Here's how the part is built. I have some questions about the finished solid (model axes, mm). A direction names the side the tool comes from. Give positions to 0.01 mm unless a question says otherwise; leave off trailing zeros. Loops run counter-clockwise (first coordinate to the right, second up) from the corner with the lowest first, then second, coordinate; pieces in that order, holes last. Notation, with made-up numbers: (27.25, -25) -> (55.25, -25) arc R28 cw to (55.25, -7) -> close; hole circle Ø9 at (2.25, 49). An arc over 180 degrees is marked (long way). Answer in a Markdown table with one row per item. Add a question column.
Item 1: We'd pull the mould along X, two halves only. Please class faces 3 (the face through (72.227, -160.39, 4.696)), 4 (the face through (124, -168, 5)), 5 (the face through (131.89, -161.88, 4.7)), 6 (the face through (31, -203.2, 5)): released by +X, released by -X, zero draft, split by the parting line, or undercut.
Item 2: If I drill on line 1 (X direction, y = -141, z = 0.5); line 2 (X direction, y = -149.5, z = 1.5); line 3 (Y direction, x = 158, z = 6.5), over which ranges is the centre line in solid material (lowest first)?
Item 3: Which directions (+Z, -Z, +X, -X, +Y, -Y) give clear straight access to the entire face, cutting with the end or side of a thin tool? Please do faces 1 (the face through (172, -203.2, 5)), 2 (the face through (80.47, -166.26, 4.7)).
Item 4: If we section it at B-B (z = 5.75): Write out the boundary of the cut face in (x, y), then the cut area to 3 significant figures.
Item 5: For P1, Ø5, axis at x = 58.5, z = 1.5, coming from the +Y side; P2, Ø3, axis at y = -185.5, z = 7, coming from the -X side, each with a flat end and sliding along its axis, tell me the tip position at first contact or that it passes through.
Item 6: If we section it at A-A (y = -196): Write out the boundary of the cut face in (x, z) (3 decimals).
Item 7: If we section it at D-D (x = 127): Write out the boundary of the cut face in (y, z) (3 decimals), then the cut area to 3 significant figures.
Item 8: If we section it at C-C (y = -183): Write out the boundary of the cut face in (x, z) (3 decimals).
Autodesk Inventor part; units mm, degrees
ref_plane "YZ Plane" through (0, 0, 0) normal (1, 0, 0) x (0, 1, 0)
ref_plane "XZ Plane" through (0, 0, 0) normal (0, 1, 0) x (-1, 0, 0)
ref_plane "XY Plane" through (0, 0, 0) normal (0, 0, 1) x (1, 0, 0)
sketch "Sketch1" plane through (0, 0, 0) normal (0, 0, 1) x (1, 0, 0)
  line L0 (0, 0) -> (203.2, 0)
  line L1 (203.2, 0) -> (203.2, -203.2)
  line L2 (0, -203.2) -> (0, 0)
  line L3 (0, -101.6) -> (203.2, -101.6)
  circle A0 centre (101.6, -101.6) radius 1.5635
  circle A1 centre (101.6, -101.6) radius 12.7
  arc A2 (26.281, -203.2) -> (88.9003, -101.509) centre (-26.321, -100.6834) ccw
  arc A3 (36.5054, -203.2) -> (101.6, -107.95) centre (-13.2987, -99.2953) ccw
  line L4 (101.6, -246.9942) -> (101.6, 0)
  arc A4 (114.2997, -101.509) -> (176.919, -203.2) centre (229.521, -100.6834) ccw
  arc A5 (101.6, -107.95) -> (166.6946, -203.2) centre (216.4987, -99.2953) ccw
  line L5 (166.6946, -203.2) -> (176.919, -203.2)
  line L6 (26.281, -203.2) -> (36.5054, -203.2)
  line L7 (0, -203.2) -> (203.2, -203.2)
  point P0 (88.9, -101.6)
  point P1 (88.8996, -101.6)
  point P2 (100.9466, -114.2832)
  point P3 (102.2534, -114.2832)
  point P4 (114.3004, -101.6)
  point P5 (114.3, -101.6)
  point P6 (171.8068, -203.2)
  point P7 (101.6, -123.4971)
  point P8 (114.2997, -101.509)
  dimension "d10" = 25.4
  dimension "d7" = 203.2
  dimension "d8" = 203.2
  dimension "d9" = 3.127
  dimension "d11" = 115.2242
  dimension "d12" = 115.2242
  dimension "d15" = 26.281
  dimension "d16" = 6.35
  dimension "d18" = 101.6
  dimension "d19" = 10.2243
extrude "Extrusion1" add sketch "Sketch1" along normal blind 9.525 contours L4 A0 L3 A1 | A1 L3 A0 L4 | L3 A0 L4 A3 A1 | A1 A3 L6 A2 | A3 L4 A1 | A1 A5 L4 A0 L3 | A4 L5 A5 A1 | L4 A5 A1
properties part number "rod support main"
Recorded:
| question | item | result |
|---|---|---|
| 1 | face 3 | released by -X |
| 1 | face 4 | undercut |
| 1 | face 5 | released by +X |
| 1 | face 6 | zero draft |
| 2 | line 1 | x = 81.62 to 94.11, 109.09 to 121.58 |
| 2 | line 2 | x = 78.05 to 90.41, 112.79 to 125.15 |
| 2 | line 3 | y = -198.57 to -191.02 |
| 3 | face 1 | +Z, -Z, +X, -X, -Y |
| 3 | face 2 | +Z, -Z, -Y |
| 4 | outline | (26.28, -203.2) -> (36.51, -203.2) arc R115.22 ccw to (100.95, -114.28) arc R12.7 ccw to (102.25, -114.28) arc R115.22 ccw to (166.69, -203.2) -> (176.92, -203.2) arc R115.22 cw to (114.3, -101.6) arc R12.7 ccw to (88.9, -101.6) arc R115.22 cw to start; hole circle Ø3.13 at (101.6, -101.6) |
| 4 | area | 2,720 mm^2 |
| 5 | P1 | stops at y = -175.86 |
| 5 | P2 | stops at x = 50.01 |
| 6 | outline | (38.42, 0) -> (49.35, 0) -> (49.35, 9.525) -> (38.42, 9.525) -> close; (153.85, 0) -> (164.78, 0) -> (164.78, 9.525) -> (153.85, 9.525) -> close |
| 7 | outline | (-171.867, 0) -> (-153.277, 0) -> (-153.277, 9.525) -> (-171.867, 9.525) -> close |
| 7 | area | 177 mm^2 |
| 8 | outline | (54.305, 0) -> (65.886, 0) -> (65.886, 9.525) -> (54.305, 9.525) -> close; (137.314, 0) -> (148.895, 0) -> (148.895, 9.525) -> (137.314, 9.525) -> close |
